The model under review builds one solid part; all positions refer to its coordinate system, in mm. Coordinates: 2 decimals unless noted, no trailing zeros. Loops run counter-clockwise (first coordinate to the right, second up) from the corner with the lowest first, then second, coordinate; pieces in that order, holes last. Notation, with made-up numbers: M -8,-19.75 L 33,-19.75 A14 ccw 33,7.25 Z; hole C 36.5,40 d7. An arc over 180 degrees is marked long. Return JSON: item names as keys, results as strings.
Autodesk Inventor part; units mm, degrees
ref_plane "YZ Plane" through (0, 0, 0) normal (1, 0, 0) x (0, 1, 0)
ref_plane "XZ Plane" through (0, 0, 0) normal (0, 1, 0) x (-1, 0, 0)
ref_plane "XY Plane" through (0, 0, 0) normal (0, 0, 1) x (1, 0, 0)
sketch "スケッチ1" plane through (0, 0, 0) normal (1, 0, 0) x (0, 1, 0)
  line L0 (0, 250) -> (88.1635, -250)
  arc A0 (0, 250) -> (88.1635, -250) centre (710.7652, 117.5543) ccw
  arc A1 (0, 250) -> (88.1635, -250) centre (325.1936, 49.5676) ccw
  line L1 (0, -370.1192) -> (0, 353.3532)
  point P0 (0, 0)
  dimension "d0" = 250
  dimension "d2" = 500
  dimension "d3" = 10
  dimension "d4" = 723
  dimension "d5" = 382
extrude "押し出し1" add sketch "スケッチ1" along normal mid plane 5 contours A0 L1 A1 | A1 L1 A0
sketch "スケッチ3" plane through (0, 0, 0) normal (1, 0, 0) x (0, 1, 0)
  circle A0 centre (-30, 128) radius 10
  circle A1 centre (-30, 0) radius 10
  circle A2 centre (20, -150) radius 10
  line L0 (-54, 0) -> (44, 0)
  line L1 (0, -219.6) -> (0, 197.6)
  point P0 (0, 0)
  dimension "d10" = 128
  dimension "d11" = 30
  dimension "d12" = 20
  dimension "d13" = 20
  dimension "d14" = 20
  dimension "d15" = 30
  dimension "d16" = 150
  dimension "d19" = 20
extrude "押し出し2" cut sketch "スケッチ3" along normal through all both and the other way through all
fillet "フィレット1" radius 10 1 edges at (0, 0, 250)
fillet "フィレット2" radius 2 1 edges at (0, 88.1635, -250)
properties part number "element_base" material "アルミニウム 6061"
1. To check wall thickness, follow line 1 (Y direction, x = -0.6, z = 0); line 2 (Z direction, x = -1.5, y = -21.5); line 3 (Y direction, x = -0.4, z = 128). State the ranges of each line that lie inside material, in increasing order.
Check values:
{"line 1": "-53.58 to -40, -20 to -2.61", "line 2": "-110.83 to -5.27, 5.27 to 122.73, 133.27 to 201.57", "line 3": "-48.67 to -40, -20 to -12.16"}
2. Add section A-A on z = 0. Give the boundary of the cut face in (x, y), plus the area to 3 significant figures.
Check values:
{"outline": "M -2.5,-53.58 L 2.5,-53.58 L 2.5,-40 L -2.5,-40 Z; M -2.5,-20 L 2.5,-20 L 2.5,-2.61 L -2.5,-2.61 Z", "area": "155 mm²"}
3. Add section C-C on x = -1.2. State how many separate pieces and enclosed holes the cut face has, plus the area to 3 significant figures.
Check values:
{"separate pieces": "1", "enclosed holes": "3", "area": "16,500 mm²"}
4. Add section B-B on z = 128. Give the boundary of the cut face in (x, y), plus the area to 3 significant figures.
Check values:
{"outline": "M -2.5,-48.67 L 2.5,-48.67 L 2.5,-40 L -2.5,-40 Z; M -2.5,-20 L 2.5,-20 L 2.5,-12.16 L -2.5,-12.16 Z", "area": "82.5 mm²"}
5. Add section D-D on y = 57. Give the boundary of the cut face in (x, z), plus the area to 3 significant figures.
Check values:
{"outline": "M -2.5,-222.45 L 2.5,-222.45 L 2.5,-191.19 L -2.5,-191.19 Z", "area": "156 mm²"}
6. The part is to be moulded in two halves that separate along Y. For faces 1 (the face through (0.04, -24.62, 136.43)), 2 (the face through (-0.035, 4.032, -34.947)), 3 (the face through (-0.035, -45.056, -44.451)), 4 (the face through (2.5, -13, -3)), say which applies: released by +Y, released by -Y, zero draft, split by the parting line, or undercut.
Check values:
{"face 1": "undercut", "face 2": "released by +Y", "face 3": "released by -Y", "face 4": "zero draft"}
7. Insertion check: pin 1 Ø1.5 at (x, z) = (0, -195) entering from +Y. The pin has a flat end and moves straight along its axis. Give the tip position at first contact, or say it passes through.
Check values:
{"pin 1": "y = 59.18"}
